Read the model definition and answer for the solid it produces. Units are mm, in the model's axes. Face numbers are marked on the shaded views. A direction names the side the tool comes from. Round coordinates to 2 decimals unless told otherwise and drop trailing zeros. Loops run counter-clockwise (first coordinate to the right, second up) from the corner with the lowest first, then second, coordinate; pieces in that order, holes last. Notation, with made-up numbers: (53, 69.5) - (81, 69.5) arc R10 cw to (81, 80.5) - close; hole circle Ø5 at (56, -21.75). An arc over 180 degrees is marked (long way). Use CSV: the item, a comma, the result in double quotes. Start each with the question number.
1. Determine the mould class of the marked faces 1, 2, 3 and 4 for opening direction Y: +Y half, -Y half, draft (parallel to the pull), parting line (faces both ways), or undercut.
2. A tool of negligible diameter and unlimited length cuts with its end or side. For the marked faces 5, 6, 7, 8 and 9, from which of +Z, -Z, +X, -X, +Y, -Y can it reach the whole face along a straight path? Write none if from no direction.
3. Given pin 1 Ø3 at (x, y) = (5, 3) entering from +Z, flat-ended and moving along its own axis, determine where the tip first touches the part or whether it passes through.
4. Consider line 1 along Z through (x, y) = (7, 2.5); line 2 along Z through (x, y) = (8.75, 2); line 3 along X through (y, z) = (9, 3.5). Determine where each line is inside the solid, lowest interval first.
5. Find section C-C (z = 9). Give the vertices of the cut face in (x, y), and give its area (3 significant figures).
6. Find section A-A (y = 8.5). Give the vertices of the cut face in (x, z), and give its area (3 significant figures).
from build123d import *

# Parameters (mm, degrees)
BOX_W           = 10
BOX_H           = 10
BOX_DEPTH       = 10
SKETCH005_R     = 2.995854
PAD_DEPTH       = 1
CHAMFER_SIZE    = 0.5
POCKET_DEPTH    = 0.1
SKETCH002_R     = 4.475809
SKETCH002_R_2   = 2.994172
POCKET001_DEPTH = 0.1
SKETCH003_R     = 4.54676
SKETCH003_R_2   = 2.980749
POCKET002_DEPTH = 0.1
SKETCH001_W     = 3.442568
SKETCH001_H     = 6.289959
POCKET003_DEPTH = 0.1
POCKET004_DEPTH = 0.1


with BuildPart() as part:
    # Box → Box (new body)
    with BuildSketch(Plane.XY):
        with Locations((5, 5)):
            Rectangle(BOX_W, BOX_H)
    extrude(amount=BOX_DEPTH)

    # Sketch005 → Pad (new body)
    with BuildSketch(Plane(origin=(0, 0, 0), x_dir=(1, 0, 0), z_dir=(0, 0, -1))):
        with Locations((5.043108, -4.966595)):
            Circle(SKETCH005_R)
    extrude(amount=PAD_DEPTH)

    # Chamfer
    chamfer_edges = [part.edges().sort_by_distance(p)[0] for p in [
        (2.047254, 4.966595, -1),
    ]]
    chamfer(chamfer_edges, length=CHAMFER_SIZE)

    # Sketch → Pocket (cut)
    with BuildSketch(Plane.XZ):
        Polygon((1.103754, 9.998665), (4.861133, 0), (9.025593, 9.981961), (8.021794, 9.981961), (4.913553, 2.531693), (2.107553, 9.998665), align=None)
        Polygon((3.302861, 9.998682), (4.959537, 5.590146), (6.798772, 9.998682), align=None)
    extrude(amount=-POCKET_DEPTH, mode=Mode.SUBTRACT)

    # Sketch002 → Pocket001 (cut)
    with BuildSketch(Plane(origin=(0, 0, 0), x_dir=(0, -1, 0), z_dir=(-1, 0, 0))):
        with Locations((-5.03441, 4.975201)):
            Circle(SKETCH002_R)
        with Locations((-5.03441, 4.975201)):
            Circle(SKETCH002_R_2, mode=Mode.SUBTRACT)
    extrude(amount=-POCKET001_DEPTH, mode=Mode.SUBTRACT)

    # Sketch003 → Pocket002 (cut)
    with BuildSketch(Plane.YZ.offset(10)):
        with Locations((4.996224, 4.975201)):
            Circle(SKETCH003_R)
        with Locations((4.996224, 4.975201)):
            Circle(SKETCH003_R_2, mode=Mode.SUBTRACT)
    extrude(amount=-POCKET002_DEPTH, mode=Mode.SUBTRACT)

    # Sketch001 → Pocket003 (cut)
    with BuildSketch(Plane.XY.offset(10)):
        Polygon((1.084873, 0), (1.084873, 8.981867), (9.042541, 8.981867), (9.042541, 0), (8.018671, 0), (8.018671, 7.807773), (2.108743, 7.807773), (2.108743, 0), align=None)
        with Locations((5.059318, 3.144979)):
            Rectangle(SKETCH001_W, SKETCH001_H)
    extrude(amount=-POCKET003_DEPTH, mode=Mode.SUBTRACT)

    # Sketch004 → Pocket004 (cut)
    with BuildSketch(Plane(origin=(0, 10, 0), x_dir=(-1, 0, 0), z_dir=(0, 1, 0))):
        Polygon((-9.031718, 0.020387), (-9.031718, 9.147731), (-1.132726, 9.147731), (-1.132726, 0.020387), (-2.177661, 0.020387), (-2.177661, 8.15491), (-7.986783, 8.15491), (-7.986783, 0.020387), align=None)
    extrude(amount=-POCKET004_DEPTH, mode=Mode.SUBTRACT)


solid = part.part
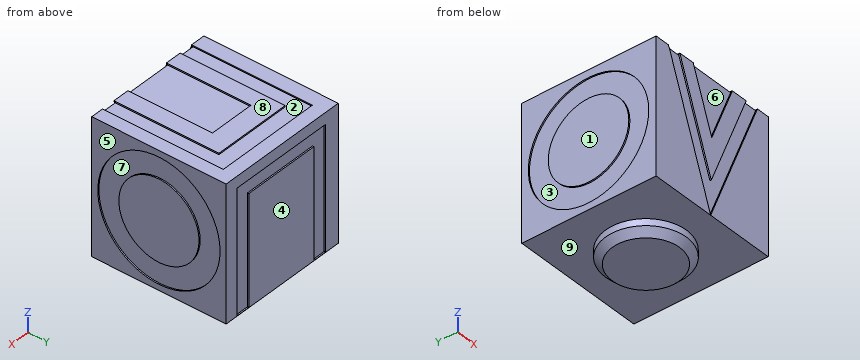
Filled sheet:
1,face 1,"draft"
1,face 2,"undercut"
1,face 3,"undercut"
1,face 4,"+Y half"
2,face 5,"+Z, -Z, +X, +Y, -Y"
2,face 6,"+Z, -Y"
2,face 7,"+X"
2,face 8,"+Z, +X, -X, +Y, -Y"
2,face 9,"-Z"
3,pin 1,"stops at z = 9.9"
4,line 1,"z = 0 to 10"
4,line 2,"z = 0 to 9.9"
4,line 3,"x = 0.1 to 9.9"
5,outline,"(0, 0) - (1.48, 0) - (1.48, 0.1) - (2.48, 0.1) - (2.48, 0) - (3.68, 0) - (3.68, 0.1) - (6.38, 0.1) - (6.38, 0) - (7.61, 0) - (7.61, 0.1) - (8.62, 0.1) - (8.62, 0) - (10, 0) - (10, 2.88) - (9.9, 2.88) - (9.9, 7.11) - (10, 7.11) - (10, 10) - (9.03, 10) - (9.03, 9.9) - (1.13, 9.9) - (1.13, 10) - (0, 10) - (0, 6.99) - (0.1, 6.99) - (0.1, 3.08) - (0, 3.08) - close"
5,area,"97.9 mm²"
6,outline,"(0, 0) - (10, 0) - (10, 2.08) - (9.9, 2.08) - (9.9, 7.87) - (10, 7.87) - (10, 10) - (9.04, 10) - (9.04, 9.9) - (1.08, 9.9) - (1.08, 10) - (0, 10) - (0, 7.81) - (0.1, 7.81) - (0.1, 2.14) - (0, 2.14) - close"
6,area,"98.1 mm²"
